For this review, take the finished solid that the model builds, in its own axes (mm). A direction names the side the tool comes from. Coordinates: 2 decimals unless noted, no trailing zeros. Order: outer loops, then holes, each group sorted by start corner. A loop starts at its lowest first (then second) coordinate and runs counter-clockwise, first axis right, second up. Notation, with made-up numbers: (0.5, -31) -> (16.5, -31) arc R28 ccw to (16.5, 7) -> close; hole circle Ø7 at (-24, 83). An arc over 180 degrees is marked (long way). Return JSON: item names as keys, results as strings. Group by question number.
Item 1: Take a section at A-A (y = 0). Write out the cut boundary in (x, z), then the cut area to 3 significant figures.
Item 2: Insertion check: pin 1 (1 mm diameter, centred on x = 100.5, y = 2, fed in from +Z); pin 2 (3 mm diameter, centred on x = 87.5, y = 5, fed in from +Z); pin 3 (4 mm diameter, centred on x = 99.5, y = 0.5, fed in from -Z). Each pin has a flat end and moves straight along its axis. Give the tip position at first contact, or say it passes through.
Item 3: For line 1 along Z through (x, y) = (15, -0.5); line 2 along Y through (x, z) = (68, -3.5); line 3 along Z through (x, y) = (39.5, 2.5), list the stretches that pass through material, from the lowest coordinate up.
Item 4: Draft analysis for pull direction Y (two halves, no side actions). For faces 3 (the flat face through (77, -6, -2)), 4 (the cylindrical face through (38.468, -3.955, 5.158)), state which applies: +Y half, -Y half, draft (parallel to the pull), parting line (faces both ways), or undercut.
Item 5: Machinability: for faces 1 (the cylindrical face through (118.44, 5.37, 1.19)), 2 (the flat face through (0, 0, 0)), which of the approach directions +Z, -Z, +X, -X, +Y, -Y give a long, thin tool a straight path to every point of the face, cutting with its end or side? Answer none if there is none.
Item 6: Take a section at D-D (x = 109). Write out the cut boundary in (y, z), then the cut area to 3 significant figures.
Item 7: Take a section at C-C (x = 29). Write out the cut boundary in (y, z).
```python
from build123d import *

# Parameters (mm, degrees)
SKETCH1_R          = 6.5
EXTRUDE1_DEPTH     = 123.5
SKETCH2_OUTSIDE_W  = 39.972
SKETCH2_OUTSIDE_H  = 39.972
SKETCH2_OUTSIDE_R  = 6
CUT_EXTRUDE1_DEPTH = 46.5
CHAMFER1_SIZE      = 1


with BuildPart() as part:
    # Sketch1 → Extrude1 (new body)
    with BuildSketch(Plane(origin=(0, 0, 0), x_dir=(0, 0, -1), z_dir=(1, 0, 0))):
        Circle(SKETCH1_R)
    extrude(amount=EXTRUDE1_DEPTH)

    # Sketch2 outside → Cut-Extrude1 (cut)
    with BuildSketch(Plane(origin=(123.5, 0, 0), x_dir=(0, 0, -1), z_dir=(1, 0, 0))):
        Rectangle(SKETCH2_OUTSIDE_W, SKETCH2_OUTSIDE_H)
        Circle(SKETCH2_OUTSIDE_R, mode=Mode.SUBTRACT)
    extrude(amount=-CUT_EXTRUDE1_DEPTH, mode=Mode.SUBTRACT)

    # Sketch3 → Cut-Revolve1 (revolve, cut)
    with BuildSketch(Plane.XY, mode=Mode.PRIVATE) as cut_revolve1_sk:
        Polygon((123.5, 10.253952542), (123.5, 5.5), (114.5, 5.5), (112.600148555, 7.399851445), (112.600148555, 10.253952542), align=None)
    revolve(cut_revolve1_sk.sketch.rotate(Axis((127.965017679, 0, 0), (-1, 0, 0)), 90), axis=Axis((127.965017679, 0, 0), (-1, 0, 0)), mode=Mode.SUBTRACT)

    # Chamfer1
    chamfer1_edges = [part.edges().sort_by_distance(p)[0] for p in [
        (0, 0, 6.5),
        (123.5, 0, 5.5),
    ]]
    chamfer(chamfer1_edges, length=CHAMFER1_SIZE)


solid = part.part
```
Findings below:
{
 "1": {"outline": "(0, -5.5) -> (1, -6.5) -> (77, -6.5) -> (77, -6) -> (114, -6) -> (114.5, -5.5) -> (122.5, -5.5) -> (123.5, -4.5) -> (123.5, 4.5) -> (122.5, 5.5) -> (114.5, 5.5) -> (114, 6) -> (77, 6) -> (77, 6.5) -> (1, 6.5) -> (0, 5.5) -> close", "area": "1,550 mm2"},
 "2": {"pin 1": "stops at z = 5.81", "pin 2": "stops at z = 4.87", "pin 3": "stops at z = -6"},
 "3": {"line 1": "z = -6.48 to 6.48", "line 2": "y = -5.48 to 5.48", "line 3": "z = -6 to 6"},
 "4": {"face 3": "draft", "face 4": "parting line"},
 "5": {"face 1": "+X", "face 2": "+Z, -Z, -X, +Y, -Y"},
 "6": {"outline": "circle Ø12 at (0, 0)", "area": "113 mm2"},
 "7": {"outline": "circle Ø13 at (0, 0)"}
}
